Autodesk Inventor part; units mm, degrees
ref_plane "YZ Plane" through (0, 0, 0) normal (1, 0, 0) x (0, 1, 0)
ref_plane "XZ Plane" through (0, 0, 0) normal (0, 1, 0) x (-1, 0, 0)
ref_plane "XY Plane" through (0, 0, 0) normal (0, 0, 1) x (1, 0, 0)
sketch "Sketch1" plane through (0, 0, 0) normal (0, 0, 1) x (1, 0, 0)
  line L0 (28, 30.2) -> (0, 30.2)
  line L1 (0, 30.2) -> (0, 0)
  line L2 (0, 15.1) -> (28, 15.1) construction
  line L3 (28, 0) -> (28, 30.2)
  line L4 (0, 0) -> (28, 0)
  line L5 (20, 15.1) -> (20, 30.2) construction
  dimension "d0" = 30.2
  dimension "d3" = 28
  dimension "d26" = 20
  dimension "d27" = 8
extrude "Extrusion1" add sketch "Sketch1" along normal blind 20
sketch "Sketch2" plane through (0, 30.2, 0) normal (0, 1, 0) x (1, 0, 0)
  line L0 (0, 0) -> (0, -20) construction
  line L1 (0, 0) -> (28, 0) construction
  line L2 (10, -10) -> (0, -10) construction
  line L3 (0, 0) -> (0, -20) construction
  dimension "d48" = 10
hole "Hole1" at (10, 30.2, 10) direction (0, -1, 0) diameter 10 end through all
sketch "Sketch3" plane through (0, 0, 0) normal (0, -1, 0) x (1, 0, 0)
  line L0 (28, 20) -> (15, 20)
  line L1 (16, 19) -> (28, 19)
  line L2 (28, 19) -> (28, 20)
  circle A0 centre (16, 20) radius 1 construction
  arc A1 (15, 20) -> (16, 19) centre (16, 20) ccw
  circle A2 centre (10, 10) radius 5 construction
  line L3 (15, 10) -> (15, 20) construction
  line L4 (0, 20) -> (28, 20) construction
  line L5 (28, 0) -> (28, 20) construction
  line L6 (10, 10) -> (15, 10) construction
  line L7 (28, 0) -> (15, 0)
  line L8 (16, 1) -> (28, 1)
  line L9 (28, 1) -> (28, 0)
  arc A3 (16, 1) -> (15, 0) centre (16, 0) ccw
  point P0 (0, 0)
  dimension "d15" = 2
  dimension "d46" = 18
extrude "Extrusion2" cut sketch "Sketch3" against normal through all
fillet "Fillet1" radius 10 2 edges at (0, 15.1, 0) (0, 15.1, 20)
sketch "Sketch4" plane through (15, 30.2, 20) normal (0, 1, 0) x (1, 0, 0)
  circle A0 centre (-5, 10) radius 5 construction
  line L0 (-5, 10) -> (13, 10) construction
  line L1 (-5, 10.9) -> (13, 10.9)
  line L2 (13, 10.9) -> (13, 9.1)
  line L3 (13, 9.1) -> (-5, 9.1)
  line L4 (-5, 9.1) -> (-5, 10.9)
  line L5 (-5, 10.9) -> (13, 9.1) construction
  line L6 (13, 10.9) -> (-5, 9.1) construction
  line L7 (13, 19) -> (13, 1) construction
  point P0 (4, 10)
  point P1 (12, 15)
  point P2 (13, 1)
  point P3 (12, 18)
  dimension "d19" = 1.8
extrude "Extrusion3" cut sketch "Sketch4" against normal through all
sketch "Sketch5" plane through (28, 0, 19) normal (1, 0, 0) x (0, 0, -1)
  circle A0 centre (9, 15.1) radius 5
  line L0 (0, 0) -> (0, 30.2) construction
  line L1 (0, 0) -> (18, 30.2) construction
  line L2 (18, 0) -> (0, 30.2) construction
  line L3 (18, 0) -> (18, 30.2) construction
  dimension "d22" = 10
extrude "Extrusion4" cut sketch "Sketch5" against normal up to surface
sketch "Sketch6" plane through (16, 0, 19) normal (0, 0, 1) x (1, 0, 0)
  line L0 (0, 30.2) -> (12, 30.2) construction
  line L1 (0, 0) -> (0, 30.2) construction
  line L2 (12, 0) -> (0, 0) construction
  line L3 (12, 30.2) -> (12, 0) construction
  line L4 (6, 0) -> (6, 30.2) construction
  line L5 (6, 15.1) -> (0, 15.1) construction
  point P0 (-16, 0)
  point P1 (6, 5.1)
  point P2 (6, 25.1)
  dimension "d28" = 10
hole "Hole2" at (22, 5.1, 19) at (22, 25.1, 19) direction (0, 0, -1) diameter 3.4 depth 8.1 counterbore diameter 6.5 counterbore depth 3.4
sketch "Sketch7" plane through (14.9183, 30.2, 9.1) normal (0, 0, 1) x (1, 0, 0)
  point P0 (-14.9183, -30.2)
  point P1 (7.0817, -5.1)
  point P2 (7.0817, -25.1)
hole "Hole3" at (22, 25.1, 9.1) at (22, 5.1, 9.1) direction (0, 0, -1) diameter 2.459 depth 8.8 tip angle 118
ref_plane "Work Plane1" through (16, 15.1, 19) normal (0, -1, 0) x (1, 0, 0)
fillet "Fillet2" radius 1 18 edges at (15.2929, 30.2, 19.2929) (22, 30.2, 19) (2.9289, 30.2, 2.9289) (12.4999, 30.2, 0) (12.4999, 30.2, 20) (15.2929, 30.2, 0.7071) (22, 30.2, 1) (15.2929, 0, 19.2929) (22, 0, 19) (12.4999, 0, 20) (12.4999, 0, 0) (2.9289, 0, 2.9289) (15.2929, 0, 0.7071) (22, 0, 1) (28, 0, 5.05) (28, 0, 14.95) (28, 30.2, 14.95) (28, 30.2, 5.05)
equation "\"d0\" = YawnFixation_Width"
equation "\"d26\" = YawnShaft_Diameter + Aufmass_ShaftFixationSide"
equation "\"d4\" = YawnShaft_Diameter + Aufmass_ShaftFixationSide"
equation "\"d48\" = 0.5 * d4"
equation "\"d7\" = YawnShaft_Diameter"
equation "\"d18\" = 0.5 * d4"
equation "\"d22\" = Shaft_DiaOut"
equation "\"Aufmass_ShaftFixationSide\" = 10"
properties part number "UpperArm_Yawn_Fixture" material "PBT Plastic"
Check sheet for the modelled part. Datum: model origin and axes. Units: mm. A direction names the side the tool comes from. Coordinates: 2 decimals unless noted, no trailing zeros. Order: outer loops, then holes, each group sorted by start corner. A loop starts at its lowest first (then second) coordinate and runs counter-clockwise, first axis right, second up. Notation, with made-up numbers: (30, -23) -> (46, -23) arc R23 ccw to (46, -4) -> close; hole circle Ø11 at (-9, 29.25). An arc over 180 degrees is marked (long way). Write item = value, one per line. Start each with the question number.
1) Cross-section at A-A (y = 5.1). State how many separate pieces and enclosed holes the cut face has, then the cut area to 3 significant figures.
2) Access from +Z, -Z, +X, -X, +Y, -Y to the whole of each face (thin tool, end or side, straight path). Record for faces 1 (the flat face through (22, 15, 1)), 2 (the cylindrical face through (21, 15, 5)), 3 (the cylindrical face through (21.916, 0.301, 1.285)).
3) Mould release check, pull along X, two halves, no side actions. Record for faces 4 (the cylindrical face through (27.699, 0.285, 5.107)), 5 (the flat face through (23.4, 23.7, 15.6)), 6 (the cylindrical face through (12.465, 0.301, 0.285)): +X half, -X half, draft (parallel to the pull), parting line (faces both ways), or undercut.
4) Go/stop test with flat-tipped pins: P1, Ø3, axis at x = 22, y = 5.1, coming from the +Z side; P2, Ø10, axis at x = 10.5, y = 3.5, coming from the -Z side; P3, Ø3.5, axis at x = 23.5, y = 14, coming from the -Z side; P4, Ø6, axis at x = 22, y = 25.1, coming from the +Z side. Record where each tip stops, or that it passes through.
5) Material ranges on L1, parallel to Y at x = 22, z = 16.45; L2, parallel to Y at x = 22, z = 3.5; L3, parallel to Z at x = 26.75, y = 24, recorded low to high.
6) Cross-section at B-B (x = 10.75). Enter the section's corners in (y, z), then the cut area to 3 significant figures.
Ans:
q1.separate_pieces = 3
q1.enclosed_holes = 0
q1.area = 332 mm²
q2.face_1 = -Z, +X, +Y, -Y
q2.face_2 = +X
q2.face_3 = -Z, +X, -Y
q3.face_4 = +X half
q3.face_5 = undercut
q3.face_6 = draft
q4.P1 = 9.1
q4.P2 = 0
q4.P3 = 1
q4.P4 = 15.6
q5.L1 = 0 to 1.85, 8.35 to 21.85, 28.35 to 30.2
q5.L2 = 0 to 3.87, 6.33 to 23.87, 26.33 to 30.2
q5.L3 = 1 to 9.1, 10.9 to 19
q6.outline = (0, 1) arc R1 ccw to (1, 0) -> (29.2, 0) arc R1 ccw to (30.2, 1) -> (30.2, 5.06) -> (15.85, 5.06) arc R5 cw to (14.35, 5.06) -> (0, 5.06) -> close; (0, 14.94) -> (14.35, 14.94) arc R5 cw to (15.85, 14.94) -> (30.2, 14.94) -> (30.2, 19) arc R1 ccw to (29.2, 20) -> (1, 20) arc R1 ccw to (0, 19) -> close
q6.area = 304 mm²
